from build123d import *

# Parameters (mm, degrees)
F0_W     = 101.6
F0_H     = 101.6
F1_DEPTH = 6.35
F2_D     = 5.1054
F3_D     = 5.1054


# Not quite as in the source:
# - a feature names something its author has since deleted; it is built from what else it names


with BuildPart() as f1:
    # F0 (on Front) → F1 (new body)
    with BuildSketch(Plane.XZ):
        Rectangle(F0_W, F0_H)
    extrude(amount=F1_DEPTH)

    # F2 (through all)
    with Locations(Plane(origin=(0, 0, 0), x_dir=(1, 0, 0), z_dir=(0, 1, 0))):
        with Locations((-38.1, -38.1), (38.1, 38.1), (-38.1, 38.1)):
            Hole(F2_D / 2)

    # F3 (through all)
    with Locations(Plane(origin=(0, 0, 0), x_dir=(1, 0, 0), z_dir=(0, 1, 0))):
        with Locations((36.6242937744, -38.9907881618)):
            Hole(F3_D / 2)


solid = f1.part
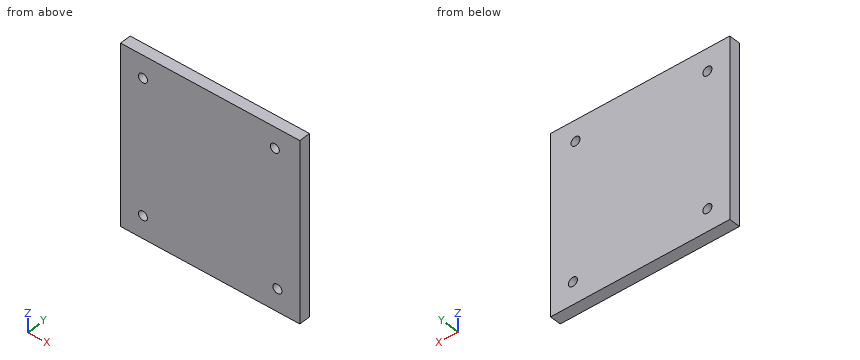
Source: CAD feature listing. Evaluate the final solid. Frame: model axes, mm. Round coordinates to 2 decimals unless told otherwise and drop trailing zeros. Loops run counter-clockwise (first coordinate to the right, second up) from the corner with the lowest first, then second, coordinate; pieces in that order, holes last. Notation, with made-up numbers: (41.5, 26) - (95.5, 26) arc R33 cw to (95.5, 59) - close; hole circle Ø3 at (-12.75, 9). An arc over 180 degrees is marked (long way). Write item = value, one per line. Start each with the question number.
(1) Section query B-B, the plane x = -38.1. Output: boundary loops of the cut face in (y, z).
(2) Ray query, line 1 along X through (y, z) = (-4, -38.1); line 2 along Z through (x, y) = (-38.5, -1). Return the intervals inside material, ascending. Write a range as from..to.
(3) Pin query (flat end, axial travel): pin 1 (4.5 mm diameter, centred on x = 36.62, z = 38.99, fed in from -Y). Return the tip coordinate at first contact, or that it passes through.
(4) Section query A-A, the plane z = -38.1. Output: boundary loops of the cut face in (x, y), plus the area to 3 significant figures.
Conclusion:
q1.outline = (-6.35, -50.8) - (0, -50.8) - (0, -40.65) - (-6.35, -40.65) - close; (-6.35, -35.55) - (0, -35.55) - (0, 35.55) - (-6.35, 35.55) - close; (-6.35, 40.65) - (0, 40.65) - (0, 50.8) - (-6.35, 50.8) - close
q2.line_1 = -50.8..-40.65, -35.55..35.55, 40.65..50.8
q2.line_2 = -50.8..-40.62, -35.58..35.58, 40.62..50.8
q3.pin_1 = through
q4.outline = (-50.8, -6.35) - (-40.65, -6.35) - (-40.65, 0) - (-50.8, 0) - close; (-35.55, -6.35) - (35.55, -6.35) - (35.55, 0) - (-35.55, 0) - close; (40.65, -6.35) - (50.8, -6.35) - (50.8, 0) - (40.65, 0) - close
q4.area = 580 mm2
